Read the model definition and answer for the solid it produces. Units are mm, in the model's axes. Give positions to 0.01 mm unless a question says otherwise; leave off trailing zeros. Write each loop counter-clockwise with the first axis right and the second up, starting at its lowest first coordinate (ties: lowest second). Pieces come first, ordered by that corner, then holes. Notation, with made-up numbers: (23, 9) -> (39, 9) arc R19 cw to (39, 25) -> close; hole circle Ø6 at (3, -32.5). An arc over 180 degrees is marked (long way). Write item = value, one per line.
from build123d import *

# Parameters (mm, degrees)
ESBO_O2_W                       = 12.7
ESBO_O2_H                       = 12.7
RESSALTO_EXTRUS_O2_DEPTH        = 75
CORTE_EXTRUS_O1_DEPTH           = 77.33225072
FURO_ROSCADO_DE_M41_D           = 3.3
FURO_ROSCADO_DE_M41_CSINK_D     = 4.05
FURO_ROSCADO_DE_M41_CSINK_ANGLE = 90


with BuildPart() as part:
    # Esboço2 → Ressalto-extrusão2 (new body)
    with BuildSketch(Plane.XY):
        Rectangle(ESBO_O2_W, ESBO_O2_H)
    extrude(amount=-RESSALTO_EXTRUS_O2_DEPTH)

    # Esboço3 → Corte-extrusão1 (cut, through all)
    with BuildSketch(Plane(origin=(6.35, 0, 0), x_dir=(0, 0, -1), z_dir=(1, 0, 0))):
        with BuildLine():
            ThreePointArc((37.5, -3.774917218), (47, 0), (37.5, 3.774917218))
            ThreePointArc((37.5, 3.774917218), (28, 0), (37.5, -3.774917218))
        make_face()
    extrude(amount=-CORTE_EXTRUS_O1_DEPTH, mode=Mode.SUBTRACT)

    # Furo roscado de M41 (through all)
    with Locations(Plane(origin=(0, 6.35, 0), x_dir=(1, 0, 0), z_dir=(0, 1, 0))):
        with Locations((0, 5.5), (0, 15.5), (0, 59.5), (0, 69.5)):
            CounterSinkHole(FURO_ROSCADO_DE_M41_D / 2, FURO_ROSCADO_DE_M41_CSINK_D / 2, counter_sink_angle=FURO_ROSCADO_DE_M41_CSINK_ANGLE)


solid = part.part
(1) The part is cut by section C-C on y = -2.5. Determine the outline of the cut face in (x, z), plus the area to 3 significant figures.
Checks:
outline = (-6.35, -75) -> (6.35, -75) -> (6.35, -46.4) -> (-6.35, -46.4) -> close; (-6.35, -28.6) -> (6.35, -28.6) -> (6.35, 0) -> (-6.35, 0) -> close; hole circle Ø3.3 at (0, -69.5); hole circle Ø3.3 at (0, -59.5); hole circle Ø3.3 at (0, -15.5); hole circle Ø3.3 at (0, -5.5)
area = 692 mm²
(2) The part is cut by section A-A on z = -41.5. Determine the outline of the cut face in (x, y), plus the area to 3 significant figures.
Checks:
outline = (-6.35, -6.35) -> (6.35, -6.35) -> (6.35, -5.5) -> (-6.35, -5.5) -> close; (-6.35, 5.5) -> (6.35, 5.5) -> (6.35, 6.35) -> (-6.35, 6.35) -> close
area = 21.6 mm²
(3) Given P1, Ø1, axis at x = -0.5, y = -1, coming from the +Z side, flat-ended and moving along its own axis, determine where the tip first touches the part or whether it passes through.
Checks:
P1 = 0
(4) The part is cut by section D-D on y = 4.5. Determine the outline of the cut face in (x, z), plus the area to 3 significant figures.
Checks:
outline = (-6.35, -75) -> (6.35, -75) -> (6.35, -44.66) -> (-6.35, -44.66) -> close; (-6.35, -38.34) -> (6.35, -38.34) -> (6.35, -36.66) -> (-6.35, -36.66) -> close; (-6.35, -30.34) -> (6.35, -30.34) -> (6.35, 0) -> (-6.35, 0) -> close; hole circle Ø3.3 at (0, -69.5); hole circle Ø3.3 at (0, -59.5); hole circle Ø3.3 at (0, -15.5); hole circle Ø3.3 at (0, -5.5)
area = 758 mm²
(5) The part is cut by section B-B on x = 0. Count the separate pieces of the cut face and the enclosed holes in it, plus the area to 3 significant figures.
Checks:
separate_pieces = 5
enclosed_holes = 1
area = 610 mm²
(6) For a pull along Z with two mould halves and no side action, classify faces 1 (the flat face through (0, 6.35, -37)), 2 (the cylindrical face through (0.4, -0.3, -3.9)), 3 (the flat face through (0, 0, 0)) as released by +Z, released by -Z, zero draft, split by the parting line, or undercut.
Checks:
face_1 = zero draft
face_2 = undercut
face_3 = released by +Z
(7) Consider L1, parallel to Y at x = 3.5, z = -41.5; L2, parallel to Z at x = 0, y = -1.5; L3, parallel to Z at x = -0.5, y = 1.25. Determine where each line is inside the solid, lowest interval first.
Checks:
L1 = -6.35 to -5.5, 5.5 to 6.35
L2 = -75 to -71.15, -67.85 to -61.15, -57.85 to -46.79, -28.21 to -17.15, -13.85 to -7.15, -3.85 to 0
L3 = -75 to -71.07, -67.93 to -61.07, -57.93 to -46.86, -28.14 to -17.07, -13.93 to -7.07, -3.93 to 0
